Job drawing, mm, ordinate dimensions from the low corner. One solid piece. Give positions to 0.01 mm unless a question says otherwise; leave off trailing zeros. Answer as a JSON object with one key per item and string values.
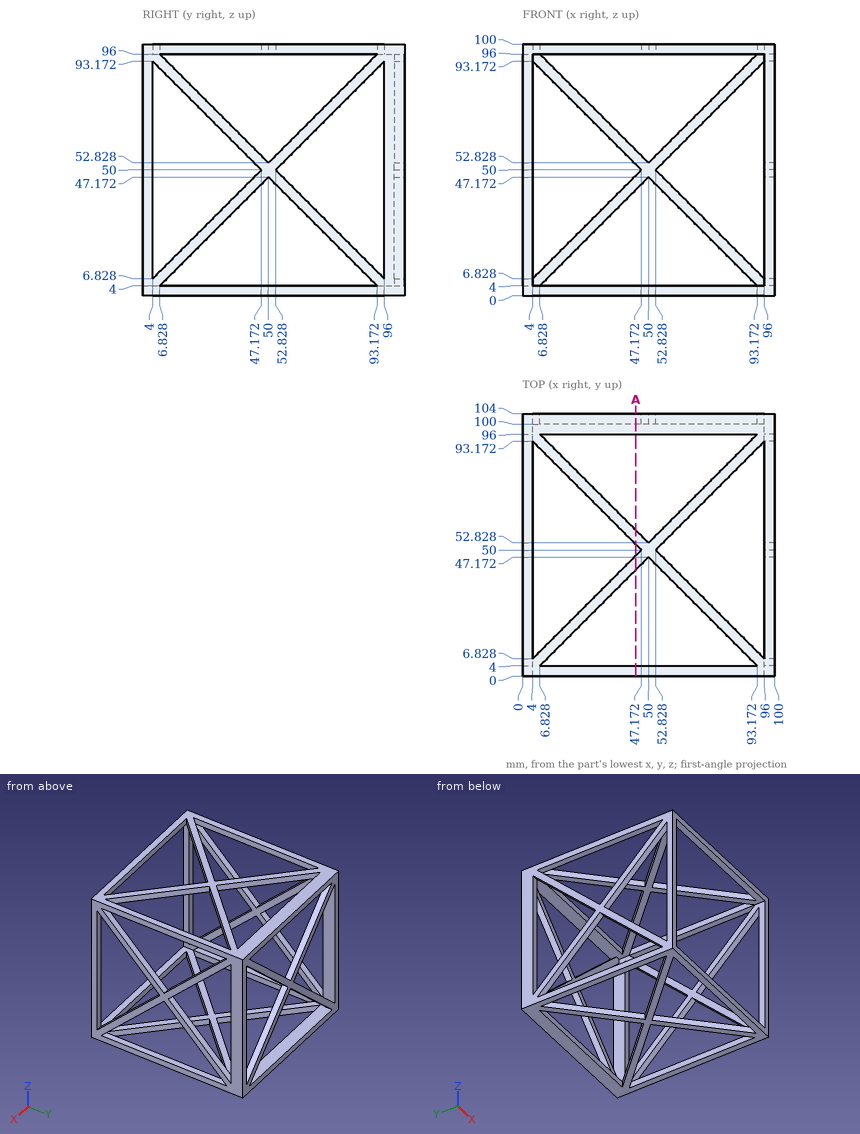
Item 1: Flat gauge pin, fed straight in: P1, Ø4, axis at x = 73.5, z = 23.5, coming from the -Y side. Where does the tip first touch, or does it go through?
Entries:
{"P1": "y = 100"}
Item 2: Cut at A-A (x = 45). State how many separate pieces and enclosed holes the cut face has, and give its area (3 significant figures).
Entries:
{"separate pieces": "10", "enclosed holes": "0", "area": "232 mm2"}
Item 3: Probe line 1 (Z direction, x = 26.5, y = 99); line 2 (Y direction, x = 96.5, z = 31.5). List the from-to ranges inside material, lowest first. Write a range as from..to.
Entries:
{"line 1": "0..4, 96..100", "line 2": "0..4, 28.67..34.33, 65.67..71.33, 96..104"}
